Here's how the part is built. I have some questions about the finished solid (model axes, mm). A direction names the side the tool comes from. Coordinates: 2 decimals unless noted, no trailing zeros. Write each loop counter-clockwise with the first axis right and the second up, starting at its lowest first coordinate (ties: lowest second). Pieces come first, ordered by that corner, then holes.
```python
from build123d import *

# Parameters (mm, degrees)
SKETCH_1_W          = 26
SKETCH_1_H          = 17
EXTRUDE_1_DEPTH     = 46
SKETCH_2_W          = 4.5
SKETCH_2_H          = 2.5
EXTRUDE_2_DEPTH     = 7.4
SKETCH_4_W          = 5
SKETCH_4_H          = 3
EXTRUDE_3_DEPTH     = 7.4
SKETCH_5_R          = 1.2
CUT_EXTRUDE_1_DEPTH = 54.114593098
CUT_EXTRUDE_2_DEPTH = 1
SKETCH_8_R          = 2.5
CUT_EXTRUDE_3_DEPTH = 4
SKETCH_9_R          = 0.975
CUT_EXTRUDE_4_DEPTH = 5
FILLET_1_R          = 0.8


with BuildPart() as part:
    # ｽｹｯﾁ1 → ﾎﾞｽ - 押し出し1 (new body)
    with BuildSketch(Plane.XY):
        Rectangle(SKETCH_1_W, SKETCH_1_H)
    extrude(amount=-EXTRUDE_1_DEPTH)

    # ｽｹｯﾁ2 → ﾎﾞｽ - 押し出し2 (add)
    with BuildSketch(Plane(origin=(13, 0, 0), x_dir=(0, 0, -1), z_dir=(1, 0, 0))):
        with Locations((12.8, -7.25)):
            Rectangle(SKETCH_2_W, SKETCH_2_H)
    extrude(amount=EXTRUDE_2_DEPTH)

    # ｽｹｯﾁ4 → ﾎﾞｽ - 押し出し3 (add)
    with BuildSketch(Plane.ZY.offset(13)):
        with Locations((-12.8, -7)):
            Rectangle(SKETCH_4_W, SKETCH_4_H)
    extrude(amount=EXTRUDE_3_DEPTH)

    # ｽｹｯﾁ5 → ｶｯﾄ - 押し出し1 (cut, through all)
    with BuildSketch(Plane(origin=(0, 8.5, 0), x_dir=(1, 0, 0), z_dir=(0, 1, 0))):
        with Locations(Location((4, 16.05, 0), (0, 0, 180))):
            Circle(SKETCH_5_R)
        with Locations(Location((-4, 16.05, 0), (0, 0, 180))):
            Circle(SKETCH_5_R)
    extrude(amount=-CUT_EXTRUDE_1_DEPTH, mode=Mode.SUBTRACT)

    # ｽｹｯﾁ6 → ｶｯﾄ - 押し出し2 (cut)
    with BuildSketch(Plane(origin=(0, 8.5, 0), x_dir=(1, 0, 0), z_dir=(0, 1, 0))):
        Polygon((-2, 19), (2, 19), (2, 25), (0.267949192, 26), (0.767949192, 26), (0.767949192, 27), (-0.767949192, 27), (-0.767949192, 26), (-0.267949192, 26), (-2, 25), align=None)
    extrude(amount=-CUT_EXTRUDE_2_DEPTH, mode=Mode.SUBTRACT)

    # ｽｹｯﾁ8 → ｶｯﾄ - 押し出し3 (cut)
    with BuildSketch(Plane(origin=(0, 8.5, 0), x_dir=(1, 0, 0), z_dir=(0, 1, 0))):
        with Locations(Location((-4, 16.05, 0), (0, 0, 180))):
            Circle(SKETCH_8_R)
        with Locations(Location((4, 16.05, 0), (0, 0, 180))):
            Circle(SKETCH_8_R)
    extrude(amount=-CUT_EXTRUDE_3_DEPTH, mode=Mode.SUBTRACT)

    # ｽｹｯﾁ9 → ｶｯﾄ - 押し出し4 (cut)
    with BuildSketch(Plane.XY):
        with Locations((-9, 4.5)):
            Circle(SKETCH_9_R)
        with Locations(Location((9, 4.5, 0), (0, 0, 180))):
            Circle(SKETCH_9_R)
    extrude(amount=-CUT_EXTRUDE_4_DEPTH, mode=Mode.SUBTRACT)

    # ﾌｨﾚｯﾄ1
    fillet_1_edges = [part.edges().sort_by_distance(p)[0] for p in [
        (16.7, -6, -10.55),
        (16.7, -8.5, -10.55),
        (16.7, -8.5, -15.05),
        (16.7, -6, -15.05),
        (20.4, -7.25, -10.55),
        (20.4, -8.5, -12.8),
        (20.4, -7.25, -15.05),
        (20.4, -6, -12.8),
        (-16.7, -8.5, -10.3),
        (-16.7, -5.5, -10.3),
        (-16.7, -5.5, -15.3),
        (-16.7, -8.5, -15.3),
        (-20.4, -7, -10.3),
        (-20.4, -5.5, -12.8),
        (-20.4, -7, -15.3),
        (-20.4, -8.5, -12.8),
    ]]
    fillet(fillet_1_edges, radius=FILLET_1_R)


solid = part.part
```
1) Imagine slicing it at D-D on x = 15. Please give me the cut outline in (y, z).
Values follow:
outline: (-8.5, -14.25) arc R0.8 ccw to (-7.7, -15.05) - (-6.8, -15.05) arc R0.8 ccw to (-6, -14.25) - (-6, -11.35) arc R0.8 ccw to (-6.8, -10.55) - (-7.7, -10.55) arc R0.8 ccw to (-8.5, -11.35) - close
2) On a 3-axis mill with a long thin cutter (end or side, diameter ignored), from which of +Z, -Z, +X, -X, +Y, -Y can I reach the whole of each face in a straight line? I mean faces 4 (the face through (-5.15, 6.53, -18.27)), 5 (the face through (16, -6, -13)), 6 (the face through (-9.974, 4.543, -2.465)). Say none if no direction works.
Values follow:
face 4: +Y
face 5: +Z, -Z, +X, +Y
face 6: +Z
3) Imagine slicing it at C-C on y = 6.25. Please give me the cut outline in (x, z).
Values follow:
outline: (-13, -46) - (13, -46) - (13, 0) - (-13, 0) - close; hole circle Ø5 at (-4, -16.05); hole circle Ø5 at (4, -16.05)
4) Will these pins go through, and if not, where does the flat tip stop? pin 1 (1.5 mm diameter, centred on x = -16, y = -7, fed in from -Z); pin 2 (1.8 mm diameter, centred on x = -9, y = 4.5, fed in from +Z); pin 3 (1.5 mm diameter, centred on y = 5.5, z = -6.5, fed in from -X); pin 4 (2 mm diameter, centred on x = -4, z = -16.05, fed in from -Y).
Values follow:
pin 1: stops at z = -15.3
pin 2: stops at z = -5
pin 3: stops at x = -13
pin 4: passes through
5) We'd pull the mould along X, two halves only. Please class faces 1 (the face through (-4.554, -1.909, -17.115)), 2 (the face through (13, 0, -23)), 3 (the face through (-13, 0, -23)): pulls with the +X half, pulls with the -X half, needs draft (parallel to the pull), parting line crosses it, or undercut.
Values follow:
face 1: undercut
face 2: pulls with the +X half
face 3: pulls with the -X half
6) I need wall thicknesses on probe 1 along Y at (x, z) = (-9, -3) (3 decimals); probe 2 along Z at (x, y) = (4, 5.4); probe 3 along Z at (x, y) = (-4, 1.5). Which ranges of each line are inside material? Lowest first, please.
Values follow:
probe 1: y = -8.5 to 3.525, 5.475 to 8.5
probe 2: z = -46 to -18.55, -13.55 to 0
probe 3: z = -46 to -17.25, -14.85 to 0
7) Imagine slicing it at A-A on x = -4. Please give me the cut outline in (y, z).
Values follow:
outline: (-8.5, -46) - (8.5, -46) - (8.5, -18.55) - (4.5, -18.55) - (4.5, -17.25) - (-8.5, -17.25) - close; (-8.5, -14.85) - (4.5, -14.85) - (4.5, -13.55) - (8.5, -13.55) - (8.5, 0) - (-8.5, 0) - close
8) Imagine slicing it at B-B on z = -16.05. Please give me the cut outline in (x, y).
Values follow:
outline: (-13, -8.5) - (-5.2, -8.5) - (-5.2, 4.5) - (-6.5, 4.5) - (-6.5, 8.5) - (-13, 8.5) - close; (-2.8, -8.5) - (2.8, -8.5) - (2.8, 4.5) - (1.5, 4.5) - (1.5, 8.5) - (-1.5, 8.5) - (-1.5, 4.5) - (-2.8, 4.5) - close; (5.2, -8.5) - (13, -8.5) - (13, 8.5) - (6.5, 8.5) - (6.5, 4.5) - (5.2, 4.5) - close
